Autodesk Inventor part; units mm, degrees
ref_plane "YZ Plane" through (0, 0, 0) normal (1, 0, 0) x (0, 1, 0)
ref_plane "XZ Plane" through (0, 0, 0) normal (0, 1, 0) x (-1, 0, 0)
ref_plane "XY Plane" through (0, 0, 0) normal (0, 0, 1) x (1, 0, 0)
sketch "Sketch1" plane through (0, 0, 0) normal (0, 1, 0) x (-1, 0, 0)
  circle A0 centre (0, 0) radius 5
  dimension "d0" = 10
extrude "Extrusion1" add sketch "Sketch1" along normal mid plane 75
sketch "Sketch2" plane through (0, 0, 0) normal (1, 0, 0) x (0, 1, 0)
  line L0 (37.5, -5) -> (37.5, 5)
  line L1 (37.5, 0) -> (37.5, 2)
  line L2 (37.5, 2) -> (37.5, -2)
  line L3 (37.5, 2) -> (-37.5, 2)
  line L4 (-37.5, 2) -> (-37.5, -2)
  line L5 (-37.5, -2) -> (37.5, -2)
  line L6 (37.5, -2) -> (37.5, 2)
  point P0 (0, 0)
  dimension "d4" = 4
  dimension "d5" = 75
sketch "Sketch3" plane through (0, 0, 0) normal (1, 0, 0) x (0, 1, 0)
  point P0 (0, 0)
extrude "Extrusion2" add sketch "Sketch2" along normal mid plane 70
sketch "Sketch4" plane through (0, 37.5, 0) normal (0, 1, 0) x (1, 0, 0)
  point P0 (0, 0)
hole "Hole1" at (0, 37.5, 0) direction (0, -1, 0) diameter 4 depth 120
properties part number "doughvpush"
Geometry: final body of the model. Coordinates: model frame, mm. A direction names the side the tool comes from. Coordinates: 2 decimals unless noted, no trailing zeros. Order: outer loops, then holes, each group sorted by start corner. A loop starts at its lowest first (then second) coordinate and runs counter-clockwise, first axis right, second up. Notation, with made-up numbers: (79, 43.5) -> (131, 43.5) arc R10 cw to (131, 49.5) -> close; hole circle Ø3 at (13.25, 19.5). An arc over 180 degrees is marked (long way). Answer in a Markdown table with one row per item.
Item 1: Section A-A on x = 0. Output: boundary loops of the cut face in (y, z), plus the area to 3 significant figures.
Return value:
| item | result |
|---|---|
| outline | (-37.5, -5) -> (37.5, -5) -> (37.5, -2) -> (-37.5, -2) -> close; (-37.5, 2) -> (37.5, 2) -> (37.5, 5) -> (-37.5, 5) -> close |
| area | 450 mm² |
Item 2: Section C-C on y = -28. Output: boundary loops of the cut face in (x, z).
Return value:
| item | result |
|---|---|
| outline | (-35, -2) -> (-4.58, -2) arc R5 ccw to (4.58, -2) -> (35, -2) -> (35, 2) -> (4.58, 2) arc R5 ccw to (-4.58, 2) -> (-35, 2) -> close; hole circle Ø4 at (0, 0) |
Item 3: Ray query, L1, parallel to X at y = -19.5, z = 0; L2, parallel to Z at x = -29.5, y = -4.5; L3, parallel to X at y = 23, z = 1.5. Return the intervals inside material, ascending.
Return value:
| item | result |
|---|---|
| L1 | x = -35 to -2, 2 to 35 |
| L2 | z = -2 to 2 |
| L3 | x = -35 to -1.32, 1.32 to 35 |
Item 4: Section D-D on x = 11. Output: boundary loops of the cut face in (y, z).
Return value:
| item | result |
|---|---|
| outline | (-37.5, -2) -> (37.5, -2) -> (37.5, 2) -> (-37.5, 2) -> close |
Item 5: Access query for faces 5 (the flat face through (-20, -1, -2)), 6 (the flat face through (20, 1, 2)), 7 (the flat face through (20, -1, -2)), 8 (the flat face through (-20, 1, 2)). Directions: +Z, -Z, +X, -X, +Y, -Y. A direction counts if a zero-diameter tool reaches every point of the face in a straight line with its end or side. Return the directions, or none.
Return value:
| item | result |
|---|---|
| face 5 | -Z, -X, +Y, -Y |
| face 6 | +Z, +X, +Y, -Y |
| face 7 | -Z, +X, +Y, -Y |
| face 8 | +Z, -X, +Y, -Y |
Item 6: Contact query for flat-ended pins moving along their axis: P1, Ø12, axis at x = 12, y = 2.5, coming from the +Z side; P2, Ø1.5, axis at x = 21.5, y = 16, coming from the -Z side; P3, Ø1.5, axis at y = 19, z = 3.5, coming from the +X side. Output: stop coordinate, or through.
Return value:
| item | result |
|---|---|
| P1 | stops at z = 2 |
| P2 | stops at z = -2 |
| P3 | stops at x = 4.18 |
Item 7: Draft query along X for faces 1 (the cylindrical face through (2, -1, 0)), 2 (the flat face through (0.5, 37.5, 2.3)), 3 (the flat face through (35, -1, 0)), 4 (the cylindrical face through (0, -1, 5)). Return one class per face: released by +X, released by -X, zero draft, split by the parting line, or undercut.
Return value:
| item | result |
|---|---|
| face 1 | undercut |
| face 2 | zero draft |
| face 3 | released by +X |
| face 4 | split by the parting line |
Item 8: Section B-B on z = 0. Output: boundary loops of the cut face in (x, y), plus the area to 3 significant figures.
Return value:
| item | result |
|---|---|
| outline | (-35, -37.5) -> (-2, -37.5) -> (-2, 37.5) -> (-35, 37.5) -> close; (2, -37.5) -> (35, -37.5) -> (35, 37.5) -> (2, 37.5) -> close |
| area | 4,950 mm² |
